Autodesk Inventor part; units mm, degrees
ref_plane "Work Plane1" through (-12.4, -4.3, -12.7) normal (1, 0, 0) x (0, 1, 0)
ref_plane "Work Plane2" through (-14.9, -3, -9.5) normal (-1, 0, 0) x (0, 0, 1)
ref_plane "YZ Plane" through (0, 0, 0) normal (1, 0, 0) x (0, 1, 0)
ref_plane "Work Plane1" through (-12.4, -4.3, -12.7) normal (1, 0, 0) x (0, 1, 0)
sketch "Sketch1" plane through (0, 0, 0) normal (1, 0, 0) x (0, 1, 0)
  line L0 (16, -9.5) -> (16, -7.1)
  line L1 (16, -9.5) -> (4, -9.5)
  line L2 (4, -9.5) -> (4, -7.1)
  line L3 (-3, -0.1) -> (4, -7.1)
  line L4 (23, -0.1) -> (-3, -0.1) construction
  line L5 (16, -7.1) -> (23, -0.1)
  line L6 (13, -7.1) -> (20, -0.1)
  line L7 (0, -0.1) -> (7, -7.1)
  line L8 (0.0414, 0) -> (1.0414, -1)
  line L9 (0.0414, 0) -> (-3, 0)
  line L10 (-3, 0) -> (-3, 2)
  line L11 (-3, 2) -> (10, 2)
  line L12 (10, -9.5) -> (10, 0) construction
  line L13 (1.0414, -1) -> (10, -1)
  line L14 (19.9586, 0) -> (18.9586, -1)
  line L15 (19.9586, 0) -> (23, 0)
  line L16 (23, 0) -> (23, 2)
  line L17 (23, 2) -> (10, 2)
  line L18 (18.9586, -1) -> (10, -1)
  point P0 (0, 0)
  dimension "d0" = 0.1
  dimension "d1" = 0.1
  dimension "d2" = 2
  dimension "d3" = 3
extrude "Extrusion1" add sketch "Sketch1" against normal up to surface (12.4 mm away)
sketch "Sketch2" plane through (-12.4, -3, 2) normal (-1, 0, 0) x (0, 0, 1)
  line L0 (-3, 21.9586) -> (-3, 4.0414)
  line L1 (-3, 4.0414) -> (-2, 3.0414)
  line L2 (-2, 3.0414) -> (-2, 0)
  line L3 (-2, 0) -> (0, 0)
  line L4 (0, 0) -> (0, 26)
  line L5 (0, 26) -> (-2, 26)
  line L6 (-2, 26) -> (-2, 22.9586)
  line L7 (-2, 22.9586) -> (-3, 21.9586)
  line L8 (0, 26) -> (0, 0)
  line L9 (-2, 0) -> (0, 0)
  line L10 (0, 0) -> (0, 26)
  line L11 (0, 26) -> (-2, 26)
  line L12 (-2, 26) -> (-2, 0)
  point P0 (-2, 3)
  point P1 (-2, 3.0414)
ref_plane "Work Plane2" through (-14.9, -3, -9.5) normal (-1, 0, 0) x (0, 0, 1)
extrude "Extrusion2" add sketch "Sketch2" along normal up to surface (2.5 mm away) contours L6 L5 L4 L3 L2 L12
mirror "Mirror1" about plane through (0, 10, 0.5) normal (1, 0, 0) of "Extrusion2", "Extrusion1"
sketch "Sketch3" plane through (-14.9, -3, 2) normal (0, 0, 1) x (1, 0, 0)
  line L0 (0, 0) -> (29.8, 0)
  line L1 (29.8, 26) -> (29.8, 0)
  line L2 (0, 26) -> (29.8, 26)
  line L3 (0, 26) -> (0, 0)
  circle A0 centre (14.9, 13) radius 1.35
  point P0 (14.9, 3)
  point P1 (0, 13)
  point P2 (14.9, 26)
  dimension "d8" = 2.7
extrude "Extrusion3" cut sketch "Sketch3" against normal through all contours A0
properties part number "hopper lid"
Can you work these out from the model? Positions are in its coordinate system, mm. A direction names the side the tool comes from. Coordinates: 2 decimals unless noted, no trailing zeros. Loops run counter-clockwise (first coordinate to the right, second up) from the corner with the lowest first, then second, coordinate; pieces in that order, holes last. Notation, with made-up numbers: (52.5, 6.5) -> (84.5, 6.5) arc R30 ccw to (84.5, 29.5) -> close; hole circle Ø9 at (54, 84). An arc over 180 degrees is marked (long way). Put each result on its own line as item: value. Start each with the question number.
Q1. I want a section at D-D (y = 14.25). Write out the boundary of the cut face in (x, z).
Q2. For faces 1 (the face through (12.4, 10.1, -0.5)), 2 (the face through (0, -2, 0)), 3 (the face through (-0.17, 0.55, -0.51)), which set-ups out of +Z, -Z, +X, -X, +Y, -Y let a thin tool reach every point of the face, with its end or its side?
Q3. I'm going to push flat-ended pins straight in: P1, Ø0.5, axis at y = 11.5, z = -0.5, coming from the -X side; P2, Ø0.5, axis at y = 5.5, z = -0.5, coming from the +X side. Where does each tip first touch, or does it pass through?
Q4. Thinking about a two-plate mould opening in X: for faces 4 (the face through (-0.176, 11.339, 0.521)), 5 (the face through (14.9, 10, 1)), 6 (the face through (-0.17, 19.45, -0.51)), 7 (the face through (-12.4, 9.9, -0.5)), which applies, pulls with the +X half, pulls with the -X half, needs draft (parallel to the pull), parting line crosses it, or undercut?
Q5. If I drill on line 1 (Y direction, x = 0, z = 0.4); line 2 (X direction, y = 1.5, z = -0.6); line 3 (Z direction, x = -5.75, y = -0.5), over which ranges is the centre line in solid material (lowest first)? Write a range as [from, to].
Q6. I want a section at C-C (x = -7). Write out the boundary of the cut face in (y, z).
Q7. I want a section at B-B (x = 0). Write out the boundary of the cut face in (y, z), plus the area to 3 significant figures.
Q8. I want a section at A-A (y = 10). Write out the boundary of the cut face in (x, z).
Taken from the geometry:
1. outline: (-14.9, 0) -> (-12.4, 0) -> (-12.4, -1) -> (12.4, -1) -> (12.4, 0) -> (14.9, 0) -> (14.9, 2) -> (-14.9, 2) -> close
2. face 1: -Z, +X, +Y, -Y
2. face 2: -Z
2. face 3: -Z, +X, -X, -Y
3. P1: stops at x = -12.4
3. P2: stops at x = 12.4
4. face 4: undercut
4. face 5: pulls with the +X half
4. face 6: needs draft
4. face 7: pulls with the -X half
5. line 1: y = [-3, 8.65], [11.35, 23]
5. line 2: x = [-12.4, 12.4]
5. line 3: z = [0, 2]
6. outline: (-3, 0) -> (0.04, 0) -> (1.04, -1) -> (18.96, -1) -> (19.96, 0) -> (23, 0) -> (23, 2) -> (-3, 2) -> close
7. outline: (-3, 0) -> (0.04, 0) -> (1.04, -1) -> (8.65, -1) -> (8.65, 2) -> (-3, 2) -> close; (11.35, -1) -> (18.96, -1) -> (19.96, 0) -> (23, 0) -> (23, 2) -> (11.35, 2) -> close
7. area: 62.8 mm2
8. outline: (-14.9, 0) -> (-12.4, 0) -> (-12.4, -1) -> (-1.35, -1) -> (-1.35, 2) -> (-14.9, 2) -> close; (1.35, -1) -> (12.4, -1) -> (12.4, 0) -> (14.9, 0) -> (14.9, 2) -> (1.35, 2) -> close
